from build123d import *

# Parameters (mm, degrees)
BOSS_EXTRUDE1_DEPTH            = 1.6
BOSS_EXTRUDE2_DEPTH            = 0.1
M2_HOLE1_FIXINGSTRUCTURE_D     = 2.4
M2_HOLE1_FIXINGSTRUCTURE_DEPTH = 200
M2_HOLE1_FIXINGSTRUCTURE_TIP   = 0.721032743
SKETCH4_R                      = 1.2
CUT_EXTRUDE1_DEPTH             = 1.7


with BuildPart() as part:
    # Sketch1 → Boss-Extrude1 (new body)
    with BuildSketch(Plane.XY):
        with BuildLine():
            Line((-31.5, 38), (-31.5, 32))
            ThreePointArc((-31.5, 32), (-31.646446609, 31.646446609), (-32, 31.5))
            Line((-32, 31.5), (-38, 31.5))
            ThreePointArc((-38, 31.5), (-38.353553391, 31.353553391), (-38.5, 31))
            Line((-38.5, 31), (-38.5, -31))
            ThreePointArc((-38.5, -31), (-38.353553391, -31.353553391), (-38, -31.5))
            Line((-38, -31.5), (-32, -31.5))
            ThreePointArc((-32, -31.5), (-31.646446609, -31.646446609), (-31.5, -32))
            Line((-31.5, -32), (-31.5, -38))
            ThreePointArc((-31.5, -38), (-31.353553391, -38.353553391), (-31, -38.5))
            Line((-31, -38.5), (31, -38.5))
            ThreePointArc((31, -38.5), (31.353553391, -38.353553391), (31.5, -38))
            Line((31.5, -38), (31.5, -32))
            ThreePointArc((31.5, -32), (31.646446609, -31.646446609), (32, -31.5))
            Line((32, -31.5), (38, -31.5))
            ThreePointArc((38, -31.5), (38.353553391, -31.353553391), (38.5, -31))
            Line((38.5, -31), (38.5, 31))
            ThreePointArc((38.5, 31), (38.353553391, 31.353553391), (38, 31.5))
            Line((38, 31.5), (32, 31.5))
            ThreePointArc((32, 31.5), (31.646446609, 31.646446609), (31.5, 32))
            Line((31.5, 32), (31.5, 38))
            ThreePointArc((31.5, 38), (31.353553391, 38.353553391), (31, 38.5))
            Line((31, 38.5), (-31, 38.5))
            ThreePointArc((-31, 38.5), (-31.353553391, 38.353553391), (-31.5, 38))
        make_face()
    extrude(amount=BOSS_EXTRUDE1_DEPTH)

    # Esboço1 → Boss-Extrude2 (add)
    with BuildSketch(Plane.XY.offset(1.6)):
        with BuildLine():
            Line((-25, -30), (25, -30))
            ThreePointArc((25, -30), (28.535533906, -28.535533906), (30, -25))
            Line((30, -25), (30, 25))
            ThreePointArc((30, 25), (28.535533906, 28.535533906), (25, 30))
            Line((25, 30), (-25, 30))
            ThreePointArc((-25, 30), (-28.535533906, 28.535533906), (-30, 25))
            Line((-30, 25), (-30, -25))
            ThreePointArc((-30, -25), (-28.535533906, -28.535533906), (-25, -30))
        make_face()
    extrude(amount=BOSS_EXTRUDE2_DEPTH)

    # M2 Hole1-FixingStructure
    with Locations(Plane(origin=(0, 0, 0), x_dir=(-1, 0, 0), z_dir=(0, 0, -1))):
        with Locations((-28, 35), (28, 35), (-28, -35), (28, -35), (35, 28), (35, -28), (-35, -28), (-35, 28)):
            Hole(M2_HOLE1_FIXINGSTRUCTURE_D / 2, depth=M2_HOLE1_FIXINGSTRUCTURE_DEPTH)
            with Locations((0, 0, -(M2_HOLE1_FIXINGSTRUCTURE_DEPTH + M2_HOLE1_FIXINGSTRUCTURE_TIP / 2))):  # 118° drill point
                Cone(0, M2_HOLE1_FIXINGSTRUCTURE_D / 2, M2_HOLE1_FIXINGSTRUCTURE_TIP, mode=Mode.SUBTRACT)

    # Sketch4 → Cut-Extrude1 (cut)
    with BuildSketch(Plane.XY.offset(1.7)):
        with Locations((-15.155444566, -8.75)):
            Circle(SKETCH4_R)
        with Locations((15.155444566, -8.75)):
            Circle(SKETCH4_R)
        with Locations((0, 17.5)):
            Circle(SKETCH4_R)
    extrude(amount=-CUT_EXTRUDE1_DEPTH, mode=Mode.SUBTRACT)


solid = part.part
Source: CAD feature listing. Evaluate the final solid. Frame: model axes, mm. A direction names the side the tool comes from. Round coordinates to 2 decimals unless told otherwise and drop trailing zeros. Order: outer loops, then holes, each group sorted by start corner. A loop starts at its lowest first (then second) coordinate and runs counter-clockwise, first axis right, second up. Notation, with made-up numbers: (77, 89) - (132, 89) arc R26 cw to (132, 121) - close; hole circle Ø9 at (-25.75, 54). An arc over 180 degrees is marked (long way). Use a Markdown table: item, result. Add a question column.
1. Mould query, pull axis X, two halves, no side actions, for faces 1 (the flat face through (0, 0, 1.7)), 2 (the cylindrical face through (-33.89, -28.46, 0.81)). Classes: +X half, -X half, draft (parallel to the pull), parting line (faces both ways), or undercut.
2. Section query D-D (z = 0.45). Give the number of separate pieces and of enclosed holes in the cut face, then the cut area to 3 significant figures.
3. Section query B-B (x = -35). Return the cut outline in (y, z), then the cut area to 3 significant figures.
4. Section query A-A (y = 17.5). Return the cut outline in (x, z).
5. Set-up query: faces 3 (the cylindrical face through (-0.26, 16.33, 0.86)), 4 (the flat face through (0, -31, 1.6)). Return all of +Z, -Z, +X, -X, +Y, -Y with unobstructed straight access to the full face (end or side cutting, diameter ignored); none if empty.
6. Line query: probe 1 along Y at (x, z) = (-28, 1.2); probe 2 along Y at (x, z) = (35, 1.15); probe 3 along Z at (x, y) = (-35, 2). Output: solid intervals per line, ascending.
7. First-contact query: pin 1 (3 mm diameter, centred on x = 28, y = -35, fed in from -Z); pin 2 (0.8 mm diameter, centred on x = -35, z = 1, fed in from +Y); pin 3 (1.9 mm diameter, centred on x = -35, y = 28, fed in from -Z); pin 4 (0.8 mm diameter, centred on x = -34.5, z = 0.5, fed in from -Y). Flat tips, straight axial feed; report the tip coordinate or a pass-through.
Derived:
| question | item | result |
|---|---|---|
| 1 | face 1 | draft |
| 1 | face 2 | undercut |
| 2 | separate pieces | 1 |
| 2 | enclosed holes | 11 |
| 2 | area | 5,680 mm2 |
| 3 | outline | (-31.5, 0) - (-29.2, 0) - (-29.2, 1.6) - (-31.5, 1.6) - close; (-26.8, 0) - (26.8, 0) - (26.8, 1.6) - (-26.8, 1.6) - close; (29.2, 0) - (31.5, 0) - (31.5, 1.6) - (29.2, 1.6) - close |
| 3 | area | 93.1 mm2 |
| 4 | outline | (-38.5, 0) - (-1.2, 0) - (-1.2, 1.7) - (-30, 1.7) - (-30, 1.6) - (-38.5, 1.6) - close; (1.2, 0) - (38.5, 0) - (38.5, 1.6) - (30, 1.6) - (30, 1.7) - (1.2, 1.7) - close |
| 5 | face 3 | +Z, -Z |
| 5 | face 4 | +Z |
| 6 | probe 1 | -38.5 to -36.2, -33.8 to 33.8, 36.2 to 38.5 |
| 6 | probe 2 | -31.5 to -29.2, -26.8 to 26.8, 29.2 to 31.5 |
| 6 | probe 3 | 0 to 1.6 |
| 7 | pin 1 | z = 0 |
| 7 | pin 2 | y = 31.5 |
| 7 | pin 3 | through |
| 7 | pin 4 | y = -31.5 |
